Design review of the part shown in the three views and the two pictorial views. Dimensions are in mm from the part's minimum x, y and z. A direction names the side the tool comes from. Round coordinates to 2 decimals unless told otherwise and drop trailing zeros. Order: outer loops, then holes, each group sorted by start corner. A loop starts at its lowest first (then second) coordinate and runs counter-clockwise, first axis right, second up. Notation, with made-up numbers: (6, -21) - (28, -21) arc R32 cw to (28, 6) - close; hole circle Ø9 at (82.5, 57). An arc over 180 degrees is marked (long way). One line per question, with ' | ' between items. Start each with the question number.
Item 1: Add section B-B on x = 42. State the section outline as (y, z) points.
Item 2: Add section C-C on y = 19.25. State the section outline as (x, z) points, and give its area (3 significant figures).
Item 3: For L1, parallel to Y at x = 31.5, z = 10.5; L2, parallel to Z at x = 7.5, y = 10.75; L3, parallel to X at y = 17, z = 11.5, list the stretches that pass through material, from the lowest coordinate up. Write a range as [from, to].
Item 4: Add section A-A on z = 11. State the section outline as (x, y) points.
Item 5: Tool access review of the marked faces 1, 2 and 3: name each direction out of +Z, -Z, +X, -X, +Y, -Y from which nothing blocks a thin tool from reaching the whole face with its end or side.
Item 6: Insertion check: pin 1 Ø8 at (x, z) = (16.5, 4.5) entering from +Y; pin 2 Ø3 at (x, z) = (13, 7) entering from -Y; pin 3 Ø1.5 at (y, z) = (21, 1.5) entering from -X; pin 4 Ø1.5 at (x, y) = (28.5, 6) entering from -Z. Each pin has a flat end and moves straight along its axis. Give the tip position at first contact, or say it passes through.
Item 7: Add section D-D on x = 32. State the section outline as (y, z) points, and give its area (3 significant figures).
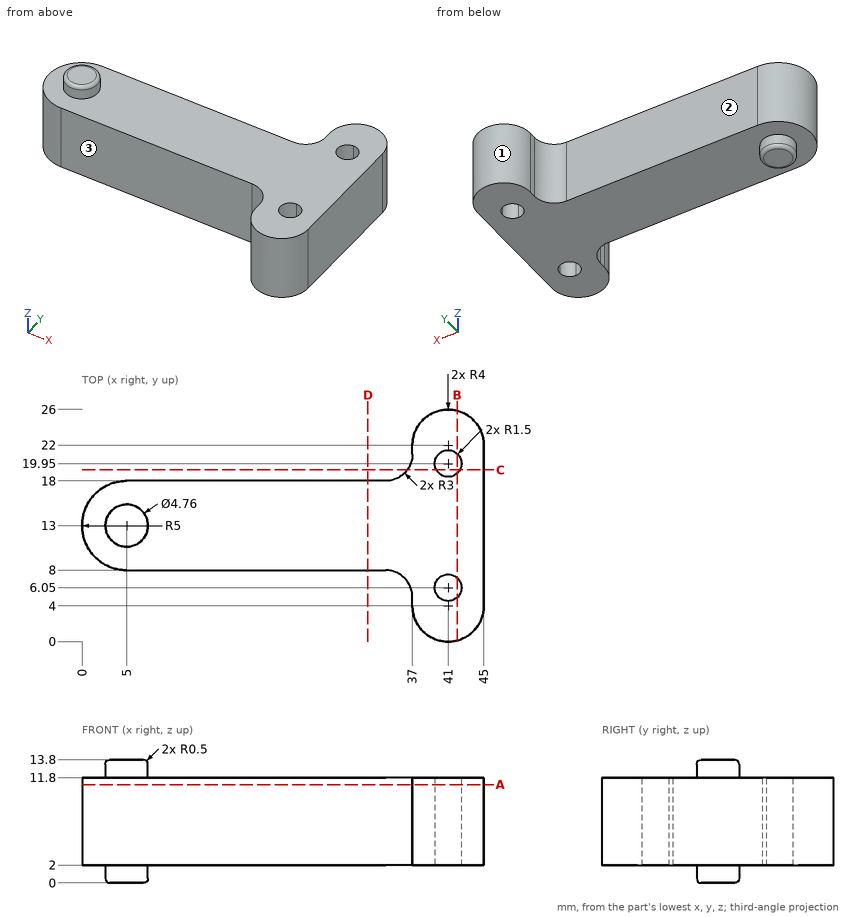
Determined:
1) outline: (0.13, 2) - (4.93, 2) - (4.93, 11.8) - (0.13, 11.8) - close; (7.17, 2) - (18.83, 2) - (18.83, 11.8) - (7.17, 11.8) - close; (21.07, 2) - (25.87, 2) - (25.87, 11.8) - (21.07, 11.8) - close
2) outline: (36.44, 2) - (39.67, 2) - (39.67, 11.8) - (36.44, 11.8) - close; (42.33, 2) - (45, 2) - (45, 11.8) - (42.33, 11.8) - close | area: 57.9 mm2
3) L1: [8, 18] | L2: [2, 11.8] | L3: [2, 45]
4) outline: (5, 8) - (34, 8) arc R3 cw to (37, 5) - (37, 4) arc R4 ccw to (45, 4) - (45, 22) arc R4 ccw to (37, 22) - (37, 21) arc R3 cw to (34, 18) - (5, 18) arc R5 ccw to start; hole circle Ø3 at (41, 6.05); hole circle Ø3 at (41, 19.95)
5) face 1: +Z, -Z, +Y | face 2: +Z, -Z, -X, +Y | face 3: +Z, -Z, -X, -Y
6) pin 1: y = 18 | pin 2: y = 8 | pin 3: x = 36.95 | pin 4: through
7) outline: (8, 2) - (18, 2) - (18, 11.8) - (8, 11.8) - close | area: 98.0 mm2
